Read the model definition and answer for the solid it produces. Units are mm, in the model's axes. A direction names the side the tool comes from. Give positions to 0.01 mm unless a question says otherwise; leave off trailing zeros. Write each loop counter-clockwise with the first axis right and the second up, starting at its lowest first coordinate (ties: lowest second). Pieces come first, ordered by that corner, then holes. Notation, with made-up numbers: (82.5, 69) - (110.5, 69) arc R25 ccw to (110.5, 92) - close; hole circle Ø2 at (36.5, 53.25). An arc over 180 degrees is marked (long way). Answer as CSV lines item,"result".
```python
from build123d import *

# Parameters (mm, degrees)
SKETCH1_W                = 82
SKETCH1_H                = 312
BOSS_EXTRUDE1_DEPTH      = 5
SKETCH2_R                = 1.25
SKETCH2_W                = 48
SKETCH2_H                = 28
CUT_EXTRUDE1_DEPTH       = 10
CHAMFER1_SIZE            = 6
FILLET1_R                = 4
SKETCH3_W                = 58
SKETCH3_H                = 68
CUT_EXTRUDE2_DEPTH       = 6
M3X0_5_TAPPED_HOLE1_D    = 2.5
FILLET2_R                = 0.5
M6_CLEARANCE_HOLE1_D     = 6.4
M6_CLEARANCE_HOLE1_DEPTH = 5
M6_CLEARANCE_HOLE1_TIP   = 1.922753981


with BuildPart() as part:
    # Sketch1 → Boss-Extrude1 (new body)
    with BuildSketch(Plane.XY):
        Rectangle(SKETCH1_W, SKETCH1_H)
    extrude(amount=BOSS_EXTRUDE1_DEPTH)

    # Sketch2 → Cut-Extrude1 (cut)
    with BuildSketch(Plane.XY.offset(5)):
        with Locations((0, -81.25)):
            Circle(SKETCH2_R)
        with Locations((0, -120.75)):
            Circle(SKETCH2_R)
        with Locations((0, -101)):
            Rectangle(SKETCH2_W, SKETCH2_H)
    extrude(amount=-CUT_EXTRUDE1_DEPTH, mode=Mode.SUBTRACT)

    # Chamfer1
    chamfer1_edges = [part.edges().sort_by_distance(p)[0] for p in [
        (24, -87, 2.5),
        (24, -115, 2.5),
    ]]
    chamfer(chamfer1_edges, length=CHAMFER1_SIZE)

    # Fillet1
    fillet1_edges = [part.edges().sort_by_distance(p)[0] for p in [
        (-24, -115, 2.5),
        (-24, -87, 2.5),
    ]]
    fillet(fillet1_edges, radius=FILLET1_R)

    # Sketch3 → Cut-Extrude2 (cut, through all)
    with BuildSketch(Plane.XY.offset(5)):
        with Locations((0, -23)):
            Rectangle(SKETCH3_W, SKETCH3_H)
    extrude(amount=-CUT_EXTRUDE2_DEPTH, mode=Mode.SUBTRACT)

    # M3x0.5 Tapped Hole1 (through all)
    with Locations(Plane.XY.offset(5)):
        with Locations((-35, 12), (35, 12), (35, -58), (-35, -58)):
            Hole(M3X0_5_TAPPED_HOLE1_D / 2)

    # Fillet2
    fillet2_edges = [part.edges().sort_by_distance(p)[0] for p in [
        (24, -93, 2.5),
        (24, -109, 2.5),
        (18, -115, 2.5),
        (18, -87, 2.5),
        (29, 11, 2.5),
        (29, -57, 2.5),
        (-29, -57, 2.5),
        (-29, 11, 2.5),
    ]]
    fillet(fillet2_edges, radius=FILLET2_R)

    # M6 Clearance Hole1
    with Locations(Plane.XY.offset(5)):
        with Locations((-26, 141), (26, 141), (-26, -141), (26, -141)):
            Hole(M6_CLEARANCE_HOLE1_D / 2, depth=M6_CLEARANCE_HOLE1_DEPTH)
            with Locations((0, 0, -(M6_CLEARANCE_HOLE1_DEPTH + M6_CLEARANCE_HOLE1_TIP / 2))):  # 118° drill point
                Cone(0, M6_CLEARANCE_HOLE1_D / 2, M6_CLEARANCE_HOLE1_TIP, mode=Mode.SUBTRACT)


solid = part.part
```
(1) A cutting plane is placed at B-B (y = 1.5). Write down the section's boundary in (x, z).
Worked out:
outline,"(-41, 0) - (-29, 0) - (-29, 5) - (-41, 5) - close; (29, 0) - (41, 0) - (41, 5) - (29, 5) - close"
(2) For faces 1 (the flat face through (21, -112, 3)), 2 (the flat face through (41, -2, 2)), determine the directions among +Z, -Z, +X, -X, +Y, -Y from which every point of the face is accessible in a straight line to the end or side of a thin tool.
Worked out:
face 1,"+Z, -Z"
face 2,"+Z, -Z, +X, +Y, -Y"
(3) A cutting plane is placed at A-A (z = 2.85). Count the separate pieces of the cut face and the enclosed holes in it, and give its area (3 significant figures).
Worked out:
separate pieces,"1"
enclosed holes,"12"
area,"20,200 mm^2"
(4) Find the intervals of material crossed by L1, parallel to Y at x = -35, z = 3.25; L2, parallel to Y at x = -10, z = 2.85; L3, parallel to Y at x = 26, z = 1.2, in increasing order.
Worked out:
L1,"y = -156 to -59.25, -56.75 to 10.75, 13.25 to 156"
L2,"y = -156 to -115, -87 to -57, 11 to 156"
L3,"y = -156 to -144.2, -137.8 to -57, 11 to 137.8, 144.2 to 156"
(5) A cutting plane is placed at D-D (x = -6.5). Write down the section's boundary in (y, z), and give its area (3 significant figures).
Worked out:
outline,"(-156, 0) - (-115, 0) - (-115, 5) - (-156, 5) - close; (-87, 0) - (-57, 0) - (-57, 5) - (-87, 5) - close; (11, 0) - (156, 0) - (156, 5) - (11, 5) - close"
area,"1,080 mm^2"
(6) A cutting plane is placed at C-C (y = -141). Write down the section's boundary in (x, z).
Worked out:
outline,"(-41, 0) - (-29.2, 0) - (-29.2, 5) - (-41, 5) - close; (-22.8, 0) - (22.8, 0) - (22.8, 5) - (-22.8, 5) - close; (29.2, 0) - (41, 0) - (41, 5) - (29.2, 5) - close"
(7) The mould has two halves that part along Y. Classify faces 3 (the flat face through (24, -101, 3)), 4 (the flat face through (-1, 156, 2)), 5 (the flat face through (-1, 37, 0)): +Y half, -Y half, draft (parallel to the pull), parting line (faces both ways), or undercut.
Worked out:
face 3,"undercut"
face 4,"+Y half"
face 5,"draft"
